The listing builds one solid part. Answer for the finished solid, in the listing's coordinates (mm). Face numbers are marked on the shaded views. A direction names the side the tool comes from. Round coordinates to 2 decimals unless told otherwise and drop trailing zeros. Order: outer loops, then holes, each group sorted by start corner. A loop starts at its lowest first (then second) coordinate and runs counter-clockwise, first axis right, second up. Notation, with made-up numbers: (9.5, -35.5) - (48.5, -35.5) arc R20 cw to (48.5, -5.5) - close; hole circle Ø5 at (43, 54.25). An arc over 180 degrees is marked (long way). Write item = value, one per line.
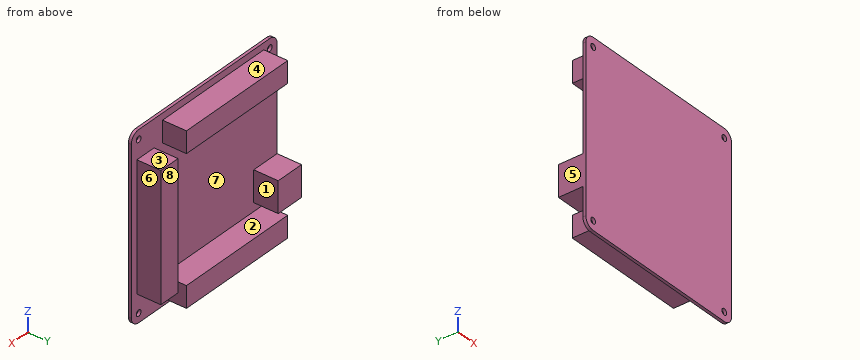
from build123d import *

# Parameters (mm, degrees)
SKETCH1_W                  = 100
SKETCH1_H                  = 100
BOSS_EXTRUDE1_DEPTH        = 1.6
FILLET1_R                  = 5
F_3_3_3_3_DIAMETER_HOLE1_D = 3.3
SKETCH4_W                  = 16
SKETCH4_H                  = 17
BOSS_EXTRUDE2_DEPTH        = 13.5
SKETCH5_W                  = 69.5
SKETCH5_H                  = 11.8
SKETCH5_W_2                = 11.8
SKETCH5_H_2                = 69.5
BOSS_EXTRUDE3_DEPTH        = 13.2


with BuildPart() as part:
    # Sketch1 → Boss-Extrude1 (new body)
    with BuildSketch(Plane(origin=(0, 0, 0), x_dir=(1, 0, 0), z_dir=(0, 1, 0))):
        Rectangle(SKETCH1_W, SKETCH1_H)
    extrude(amount=BOSS_EXTRUDE1_DEPTH)

    # Fillet1
    fillet1_edges = [part.edges().sort_by_distance(p)[0] for p in [
        (50, 0.8, 50),
        (-50, 0.8, 50),
        (-50, 0.8, -50),
        (50, 0.8, -50),
    ]]
    fillet(fillet1_edges, radius=FILLET1_R)

    # Ø3.3 (3.3) Diameter Hole1 (through all)
    with Locations(Plane(origin=(0, 1.6, 0), x_dir=(1, 0, 0), z_dir=(0, 1, 0))):
        with Locations((45, -45), (-45, -45), (-45, 45), (45, 45)):
            Hole(F_3_3_3_3_DIAMETER_HOLE1_D / 2)

    # Sketch4 → Boss-Extrude2 (add)
    with BuildSketch(Plane(origin=(0, 1.6, 0), x_dir=(1, 0, 0), z_dir=(0, 1, 0))):
        with Locations((-42, 20.7)):
            Rectangle(SKETCH4_W, SKETCH4_H)
    extrude(amount=BOSS_EXTRUDE2_DEPTH)

    # Sketch5 → Boss-Extrude3 (add)
    with BuildSketch(Plane(origin=(0, 1.6, 0), x_dir=(1, 0, 0), z_dir=(0, 1, 0))):
        with Locations((-6.15, 39.7)):
            Rectangle(SKETCH5_W, SKETCH5_H)
        with Locations((40.3, -0.25)):
            Rectangle(SKETCH5_W_2, SKETCH5_H_2)
        with Locations((-6.15, -40.4)):
            Rectangle(SKETCH5_W, SKETCH5_H)
    extrude(amount=BOSS_EXTRUDE3_DEPTH)


solid = part.part
Q1. Section B-B on x = -23 is taken. Determine the outline of the cut face in (y, z).
Model answer:
outline = (0, -50) - (1.6, -50) - (1.6, -45.6) - (14.8, -45.6) - (14.8, -33.8) - (1.6, -33.8) - (1.6, 34.5) - (14.8, 34.5) - (14.8, 46.3) - (1.6, 46.3) - (1.6, 50) - (0, 50) - close
Q2. Find the intervals of material crossed by line 1 (X direction, y = 1.2, z = 45); line 2 (X direction, y = 8.5, z = -23.5), in increasing order. Write a range as from..to.
Model answer:
line_1 = -50..-46.65, -43.35..43.35, 46.65..50
line_2 = -50..-34, 34.4..46.2
Q3. For the marked faces 1, 2, 3, 4 and 5, determine the directions among +Z, -Z, +X, -X, +Y, -Y from which every point of the face is accessible in a straight line to the end or side of a thin tool.
Model answer:
face_1 = +Y
face_2 = -X, +Y
face_3 = +Z, +X, +Y
face_4 = +Z, +X, -X, +Y
face_5 = +Z, -Z, -X, +Y, -Y
Q4. Section D-D on z = -21 is taken. Determine the outline of the cut face in (x, y), then the cut area to 3 significant figures.
Model answer:
outline = (-50, 0) - (50, 0) - (50, 1.6) - (46.2, 1.6) - (46.2, 14.8) - (34.4, 14.8) - (34.4, 1.6) - (-34, 1.6) - (-34, 15.1) - (-50, 15.1) - close
area = 532 mm^2
Q5. Section C-C on z = -5 is taken. Determine the outline of the cut face in (x, y).
Model answer:
outline = (-50, 0) - (50, 0) - (50, 1.6) - (46.2, 1.6) - (46.2, 14.8) - (34.4, 14.8) - (34.4, 1.6) - (-50, 1.6) - close
Q6. Determine the mould class of the marked faces 6, 7 and 8 for opening direction X: released by +X, released by -X, zero draft, split by the parting line, or undercut.
Model answer:
face_6 = released by +X
face_7 = undercut
face_8 = zero draft
Q7. Section A-A on y = 11.5 is taken. Determine the outline of the cut face in (x, z).
Model answer:
outline = (-50, -29.2) - (-34, -29.2) - (-34, -12.2) - (-50, -12.2) - close; (-40.9, -45.6) - (28.6, -45.6) - (28.6, -33.8) - (-40.9, -33.8) - close; (-40.9, 34.5) - (28.6, 34.5) - (28.6, 46.3) - (-40.9, 46.3) - close; (34.4, -34.5) - (46.2, -34.5) - (46.2, 35) - (34.4, 35) - close
Q8. Flat-ended cylindrical pins translate along their axes: P1, Ø7, axis at y = 8.5, z = -21, coming from the +X side; P2, Ø2, axis at x = 18, z = 12, coming from the +Y side; P3, Ø5, axis at x = 11, y = 10.5, coming from the +Z side. Find the tip coordinate at first contact, or state that the pin passes through.
Model answer:
P1 = 46.2
P2 = 1.6
P3 = 46.3
